Autodesk Fusion 360 part; units mm, degrees
sketch "Sketch1" plane through (0, 0, 0) normal (0, 0, 1) x (1, 0, 0) in component "Component"
  line L0 (12.5, -10) -> (-12.5, -10)
  line L1 (-12.5, -10) -> (-12.5, 10)
  line L2 (-12.5, 10) -> (12.5, 10)
  line L3 (12.5, 10) -> (12.5, -10)
  line L4 (12.5, -10) -> (-12.5, 10) construction
  line L5 (-12.5, -10) -> (12.5, 10) construction
  line L6 (-12.5, 0) -> (12.5, 0) construction
  line L7 (0, 10) -> (0, -10) construction
  circle A0 centre (-8.25, 0) radius 1.7
  circle A1 centre (6.25, 0) radius 2.7
  dimension "d7" = 25
  dimension "d8" = 20
  dimension "d9" = 3.4
  dimension "d10" = 5.4
  dimension "d11" = 4.25
  dimension "d12" = 6.25
extrude "Extrude1" add sketch "Sketch1" along normal mid plane 5.6 in component "Component"
fillet "Fillet1" radius 3 4 edges at (-12.5, -10, 0) (12.5, -10, 0) (12.5, 10, 0) (-12.5, 10, 0) in component "Component"
chamfer "Chamfer1" distance 0.4 angle 45 12 edges at (0, -10, 2.8) (11.6213, -9.1213, 2.8) (12.5, 0, 2.8) (11.6213, 9.1213, 2.8) (0, 10, 2.8) (-11.6213, 9.1213, 2.8) (-12.5, 0, 2.8) (-11.6213, -9.1213, 2.8) (3.7327, 0.9764, 2.8) (-9.835, 0.6147, 2.8) (3.7327, -0.9764, -2.8) (-9.835, -0.6147, -2.8) in component "Component"
sketch "Sketch2" plane through (0, 0, 2.8) normal (0, 0, 1) x (-1, 0, 0) in component "Component"
  circle A0 centre (-6.25, 0) radius 3.1
  line L0 (9.5, 9.6) -> (-9.5, 9.6)
  arc A1 (-9.5, 9.6) -> (-12.1, 7) centre (-9.5, 7) ccw
  line L1 (-12.1, 7) -> (-12.1, -7)
  arc A2 (-12.1, -7) -> (-9.5, -9.6) centre (-9.5, -7) ccw
  line L2 (-9.5, -9.6) -> (9.5, -9.6)
  arc A3 (9.5, -9.6) -> (12.1, -7) centre (9.5, -7) ccw
  line L3 (12.1, -7) -> (12.1, 7)
  arc A4 (12.1, 7) -> (9.5, 9.6) centre (9.5, 7) ccw
  circle A5 centre (8.25, 0) radius 2.1
  line L4 (12.5, -10) -> (-12.5, -10)
  line L5 (12.5, 10) -> (12.5, -10)
  line L6 (-12.5, 10) -> (12.5, 10)
  line L7 (-12.5, -10) -> (-12.5, 10)
  line L8 (6.1, -10) -> (-3.1, -10)
  line L9 (-3.1, -10) -> (-3.1, 10)
  line L10 (-3.1, 10) -> (6.1, 10)
  line L11 (6.1, 10) -> (6.1, -10)
  dimension "d19" = 9.4
  dimension "d28" = 9.2
extrude "Extrude2" cut sketch "Sketch2" against normal blind 0.6 contours L0 L2 L9 L11 | L0 L6 L9 L10 L11 | L2 L4 L8 L9 L11 in component "Component"
sketch "Sketch3" plane through (0, 0, 2.8) normal (0, 0, 1) x (-1, 0, 0) in component "Component"
  line L0 (-3.1, -9.6) -> (-3.1, 9.6)
  line L1 (-3.1, 9.6) -> (-9.5, 9.6)
  arc A0 (-9.5, 9.6) -> (-12.1, 7) centre (-9.5, 7) ccw
  line L2 (-12.1, 7) -> (-12.1, -7)
  arc A1 (-12.1, -7) -> (-9.5, -9.6) centre (-9.5, -7) ccw
  line L3 (-9.5, -9.6) -> (-3.1, -9.6)
  circle A2 centre (-6.25, 0) radius 3.1
  line L4 (12.5, -10) -> (-12.5, -10)
  line L5 (12.5, 10) -> (12.5, -10)
  line L6 (-12.5, 10) -> (12.5, 10)
  line L7 (-12.5, -10) -> (-12.5, 10)
  line L8 (-8, 1.5) -> (8, 1.5)
  line L9 (8, 1.5) -> (8, -1.5)
  line L10 (8, -1.5) -> (-8, -1.5)
  line L11 (-8, -1.5) -> (-8, 1.5)
  line L12 (-8, 1.5) -> (8, -1.5) construction
  line L13 (8, 1.5) -> (-8, -1.5) construction
  dimension "d22" = 3
  dimension "d23" = 16
extrude "Extrude3" cut sketch "Sketch3" against normal blind 0.6 contours L0 A2 L8 L10 | L0 L8 L9 L10 | A2 L8 L10 L11 picked at (-6.3833, 0) in component "Component"
component "Component" placed x (1, 0, 0) y (0, 1, 0) z (0, 0, 1) at (0, 0, 0)
equation "d7 = z_belt_width + 16 mm"
equation "d13 = ( 5.6 / 2 ) * 1 mm"
equation "d17 = chamfer"
equation "z_belt_width = 9 mm"
equation "tolerance = 0.2 mm"
equation "d28 = z_belt_width + tolerance"
equation "chamfer = 0.4 mm"
CAD build for the part. Positions are in the model's coordinates, mm. Give positions to 0.01 mm unless a question says otherwise; leave off trailing zeros. Loops run counter-clockwise (first coordinate to the right, second up) from the corner with the lowest first, then second, coordinate; pieces in that order, holes last. Notation, with made-up numbers: M -39,78 L -32,78 A14 ccw -32,105 Z; hole C 0.5,-29.75 d2. An arc over 180 degrees is marked long. Answer in a Markdown table with one row per item. Add a question column.
Item 1: Drop flat-ended pins along their axis: P1, Ø0.5, axis at x = 3.5, z = 2.5, coming from the -Y side; P2, Ø3, axis at x = -8.25, y = 0, coming from the -Z side; P3, Ø5.5, axis at x = -3, y = -3, coming from the +Z side. Give the stop position or say it passes through.
Item 2: Probe probe 1 along Y at (x, z) = (-8.25, 0.7); probe 2 along X at (y, z) = (1.5, -0.35) (3 decimals); probe 3 along X at (y, z) = (0.5, 0.85). List the from-to ranges inside material, lowest first.
Item 3: Mould opens along Y. For faces 1 (the face through (-12.5, 0, 0)), 2 (the face through (-11.6, -9.14, -0.24)), 3 (the face through (8.825, -0.811, -0.034)), 4 (the face through (0, 10, 0)) say: +Y half, -Y half, draft (parallel to the pull), parting line (faces both ways), or undercut.
Item 4: Band-saw the part on A-A on x = -8.25. Give the cut face in (y, z).
Item 5: Band-saw the part on B-B on y = 0. Give the cut face in (x, z), then the cut area to 3 significant figures.
Item 6: Band-saw the part on D-D on y = 4.75. Give the cut face in (x, z), then the cut area to 3 significant figures.
Item 7: Band-saw the part on C-C on z = 0.25. Give the cut face in (x, y), then the cut area to 3 significant figures.
Reply:
| question | item | result |
|---|---|---|
| 1 | P1 | stops at y = -10 |
| 1 | P2 | passes through |
| 1 | P3 | stops at z = 2.2 |
| 2 | probe 1 | y = -10 to -1.7, 1.7 to 10 |
| 2 | probe 2 | x = -12.5 to -9.05, -7.45 to 4.005, 8.495 to 12.5 |
| 2 | probe 3 | x = -12.5 to -9.87, -6.63 to 3.6, 8.9 to 12.5 |
| 3 | face 1 | draft |
| 3 | face 2 | -Y half |
| 3 | face 3 | undercut |
| 3 | face 4 | +Y half |
| 4 | outline | M -10,-2.8 L -2.1,-2.8 L -1.7,-2.4 L -1.7,2.4 L -2.1,2.8 L -9.6,2.8 L -10,2.4 Z; M 1.7,-2.4 L 2.1,-2.8 L 10,-2.8 L 10,2.4 L 9.6,2.8 L 2.1,2.8 L 1.7,2.4 Z |
| 5 | outline | M -12.5,-2.8 L -10.35,-2.8 L -9.95,-2.4 L -9.95,2.4 L -10.35,2.8 L -12.1,2.8 L -12.5,2.4 Z; M -6.55,-2.4 L -6.15,-2.8 L 3.15,-2.8 L 3.55,-2.4 L 3.55,2.2 L -6.55,2.2 Z; M 8.95,-2.4 L 9.35,-2.8 L 12.5,-2.8 L 12.5,2.4 L 12.1,2.8 L 9.35,2.8 L 8.95,2.4 Z |
| 5 | area | 84.0 mm^2 |
| 6 | outline | M -12.5,-2.8 L 12.5,-2.8 L 12.5,2.4 L 12.1,2.8 L 3.1,2.8 L 3.1,2.2 L -6.1,2.2 L -6.1,2.8 L -12.1,2.8 L -12.5,2.4 Z |
| 6 | area | 134 mm^2 |
| 7 | outline | M -12.5,-7 A3 ccw -9.5,-10 L 9.5,-10 A3 ccw 12.5,-7 L 12.5,7 A3 ccw 9.5,10 L -9.5,10 A3 ccw -12.5,7 Z; hole C -8.25,0 d3.4; hole C 6.25,0 d5.4 |
| 7 | area | 460 mm^2 |
